Check sheet for the modelled part. Datum: model origin and axes. Units: mm. A direction names the side the tool comes from. Coordinates: 2 decimals unless noted, no trailing zeros. Order: outer loops, then holes, each group sorted by start corner. A loop starts at its lowest first (then second) coordinate and runs counter-clockwise, first axis right, second up.
1. Set-up check for faces 1 (the flat face through (-80, -3, 38)), 2 (the flat face through (150, -3, 161)), 3 (the flat face through (80, -3, 37)), 4 (the cylindrical face through (-0.651, 194.93, 170.066)): record each of +Z, -Z, +X, -X, +Y, -Y from which the full face is reachable in a straight line by a thin tool's end or side.
2. Cross-section at A-A (y = 32). Enter the section's corners in (x, z), then the cut area to 3 significant figures.
3. Thickness scan on line 1 (Y direction, x = -46, z = 83); line 2 (X direction, y = -6.5, z = 38); line 3 (Z direction, x = -103, y = -110). Record the ranges inside material, lowest first.
4. Draft check along X on faces 5 (the flat face through (0, 200, 175)), 6 (the cylindrical face through (-0.651, -195.07, 170.066)), 7 (the cylindrical face through (115.962, -2.66, 63.438)). Enter one of: released by +X, released by -X, zero draft, split by the parting line, or undercut.
5. Cross-section at D-D (z = 34). Enter the section's corners in (x, y), then the cut area to 3 significant figures.
6. Gauge pin test, flat ends, axial feed: pin 1 Ø2 at (x, z) = (90.5, 63.5) entering from -Y; pin 2 Ø5 at (x, z) = (-73.5, 217) entering from +Y; pin 3 Ø2 at (y, z) = (102, 68) entering from -X. Record the tip position at first contact, or that the pin passes through.
7. Cross-section at B-B (x = 0). Enter the section's corners in (y, z), then the cut area to 3 significant figures.
8. Cross-section at C-C (z = 199). Enter the section's corners in (x, y), then the cut area to 3 significant figures.
```python
from build123d import *

# Parameters (mm, degrees)
SKETCH1_W           = 340
SKETCH1_H           = 400
BOSS_EXTRUDE1_DEPTH = 240
CAVITY2_START       = -200
CAVITY2_DEPTH       = 400
CAVITY2_2_OUTLINE_R = 5
CAVITY2_2_DEPTH     = 10
CAVITY2_START_2     = 190
CAVITY2_3_OUTLINE_R = 5
CAVITY2_3_DEPTH     = 10


# Read off the part's stored shape, not the designer's step: Cavity2
with BuildPart() as part:
    # Sketch1 → Boss-Extrude1 (new body)
    with BuildSketch(Plane.XY):
        Rectangle(SKETCH1_W, SKETCH1_H)
    extrude(amount=BOSS_EXTRUDE1_DEPTH)

    # Cavity2 outline → Cavity2 (cut)
    with BuildSketch(Plane(origin=(0, 0, 0), x_dir=(1, 0, 0), z_dir=(0, 1, 0)).offset(CAVITY2_START)):
        with BuildLine():
            Line((-80, -48.123427946), (-80, -27.108908401))
            ThreePointArc((-80, -27.108908401), (0, -15.02389766), (80, -27.108908401))
            Line((80, -27.108908401), (80, -48.123427946))
            ThreePointArc((80, -48.123427946), (116.45426588, -63.695656752), (150, -84.816535832))
            Line((150, -84.816535832), (150, -240))
            Line((150, -240), (170, -240))
            Line((170, -240), (170, 0))
            Line((170, 0), (-170, 0))
            Line((-170, 0), (-170, -240))
            Line((-170, -240), (-150, -240))
            Line((-150, -240), (-150, -84.816535832))
            ThreePointArc((-150, -84.816535832), (-116.45426588, -63.695656752), (-80, -48.123427946))
        make_face()
    extrude(amount=CAVITY2_DEPTH, mode=Mode.SUBTRACT)

    # Cavity2 2 outline → Cavity2 2 (cut)
    with BuildSketch(Plane(origin=(0, 0, 0), x_dir=(1, 0, 0), z_dir=(0, 1, 0)).offset(CAVITY2_START)):
        with BuildLine():
            ThreePointArc((80, -27.108908401), (0, -15.02389766), (-80, -27.108908401))
            Line((-80, -27.108908401), (-80, -48.123427946))
            ThreePointArc((-80, -48.123427946), (-116.45426588, -63.695656752), (-150, -84.816535832))
            Line((-150, -84.816535832), (-150, -240))
            Line((-150, -240), (150, -240))
            Line((150, -240), (150, -84.816535832))
            ThreePointArc((150, -84.816535832), (116.45426588, -63.695656752), (80, -48.123427946))
            Line((80, -48.123427946), (80, -27.108908401))
        make_face()
        with Locations((0, -175.02389766)):
            Circle(CAVITY2_2_OUTLINE_R, mode=Mode.SUBTRACT)
    extrude(amount=CAVITY2_2_DEPTH, mode=Mode.SUBTRACT)

    # Cavity2 3 outline → Cavity2 3 (cut)
    with BuildSketch(Plane(origin=(0, 0, 0), x_dir=(1, 0, 0), z_dir=(0, 1, 0)).offset(CAVITY2_START_2)):
        with BuildLine():
            ThreePointArc((80, -27.108908401), (0, -15.02389766), (-80, -27.108908401))
            Line((-80, -27.108908401), (-80, -48.123427946))
            ThreePointArc((-80, -48.123427946), (-116.45426588, -63.695656752), (-150, -84.816535832))
            Line((-150, -84.816535832), (-150, -240))
            Line((-150, -240), (150, -240))
            Line((150, -240), (150, -84.816535832))
            ThreePointArc((150, -84.816535832), (116.45426588, -63.695656752), (80, -48.123427946))
            Line((80, -48.123427946), (80, -27.108908401))
        make_face()
        with Locations((0, -175.02389766)):
            Circle(CAVITY2_3_OUTLINE_R, mode=Mode.SUBTRACT)
    extrude(amount=CAVITY2_3_DEPTH, mode=Mode.SUBTRACT)


solid = part.part
```
Data:
1. face 1: -Z, -X, +Y, -Y
1. face 2: +Z, -Z, +X, +Y, -Y
1. face 3: -Z, +X, +Y, -Y
1. face 4: +Y
2. outline: (-150, 84.82) arc R250.83 ccw to (-80, 48.12) - (-80, 27.11) arc R270.83 ccw to (80, 27.11) - (80, 48.12) arc R250.83 ccw to (150, 84.82) - (150, 240) - (-150, 240) - close
2. area: 60,000 mm2
3. line 1: y = -190 to 190
3. line 2: x = -80 to 80
3. line 3: z = 57.15 to 240
4. face 5: zero draft
4. face 6: split by the parting line
4. face 7: released by +X
5. outline: (-80, -190) - (80, -190) - (80, 190) - (-80, 190) - close
5. area: 60,800 mm2
6. pin 1: stops at y = -190
6. pin 2: stops at y = 190
6. pin 3: stops at x = -126.06
7. outline: (-200, 170.02) - (-190, 170.02) - (-190, 15.02) - (190, 15.02) - (190, 170.02) - (200, 170.02) - (200, 180.02) - (190, 180.02) - (190, 240) - (-190, 240) - (-190, 180.02) - (-200, 180.02) - close
7. area: 85,700 mm2
8. outline: (-150, -190) - (150, -190) - (150, 190) - (-150, 190) - close
8. area: 114,000 mm2
